The listing builds one solid part. Answer for the finished solid, in the listing's coordinates (mm). A direction names the side the tool comes from. Round coordinates to 2 decimals unless told otherwise and drop trailing zeros. Write each loop counter-clockwise with the first axis right and the second up, starting at its lowest first coordinate (ties: lowest second). Pieces come first, ordered by that corner, then holes.
Item 1: Find section B-B on y = 2.75. Give the vertices of the cut face in (x, z).
Item 2: Find the intervals of material crossed by probe 1 along X at (y, z) = (8.25, 0); probe 2 along Z at (x, y) = (-9.25, 2.75); probe 3 along Y at (x, z) = (9.75, 0), in increasing order.
Item 3: Find section C-C on z = -1.25. Give the vertices of the cut face in (x, y), then the cut area to 3 significant figures.
Item 4: Find section D-D on x = -10.5. Give the vertices of the cut face in (y, z), then the cut area to 3 significant figures.
Item 5: Find section A-A on x = 0. Give the vertices of the cut face in (y, z), then the cut area to 3 significant figures.
Item 6: A tool of negligible diameter and unlimited length cuts with its end or side. For faces 4 (the face through (-8, 5, 3)), 5 (the face through (8, 5, 3)), 6 (the face through (8, 5, -3)), 7 (the face through (0.1, 2.5, -2.5)), 8 (the face through (-8, 5, -3)), from which of +Z, -Z, +X, -X, +Y, -Y can it reach the whole face along a straight path? Write none if from no direction.
Item 7: For a pull along Y with two mould halves and no side action, classify faces 1 (the face through (-7.363, 4.485, 0.228)), 2 (the face through (-1, 7, 0)), 3 (the face through (0, 9.5, 2)) as +Y half, -Y half, draft (parallel to the pull), parting line (faces both ways), or undercut.
Item 8: Each of these flat-tipped pins is pushed along its axis until it touches: pin 1 (2 mm diameter, centred on x = -9, z = -3, fed in from -Y); pin 2 (4 mm diameter, centred on x = -9, y = 5, fed in from +Z); pin 3 (2.5 mm diameter, centred on x = 0, z = 0, fed in from -Y). Where does it stop, or does it pass through?
```python
from build123d import *

# Parameters (mm, degrees)
SKETCH1_R           = 4.7
SKETCH1_R_2         = 2.5
BOSS_EXTRUDE1_DEPTH = 5
SKETCH2_R           = 4.7
BOSS_EXTRUDE2_DEPTH = 4.5
SKETCH3_R           = 1
CUT_EXTRUDE1_DEPTH  = 4.5
SKETCH6_W           = 6
SKETCH6_H           = 6
BOSS_EXTRUDE3_DEPTH = 8.31
SKETCH7_W           = 6
SKETCH7_H           = 6
BOSS_EXTRUDE4_DEPTH = 2
FILLET1_R           = 1
BOSS_EXTRUDE5_DEPTH = 3
BOSS_EXTRUDE6_DEPTH = 9
FILLET2_R           = 1
SKETCH8_R           = 1.75
CUT_EXTRUDE6_DEPTH  = 37


with BuildPart() as part:
    # Sketch1 → Boss-Extrude1 (new body)
    with BuildSketch(Plane(origin=(0, 0, 0), x_dir=(1, 0, 0), z_dir=(0, 1, 0))):
        with Locations(Location((0, 0, 0), (0, 0, 270))):
            Circle(SKETCH1_R)
        with Locations(Location((0, 0, 0), (0, 0, 270))):
            Circle(SKETCH1_R_2, mode=Mode.SUBTRACT)
    extrude(amount=BOSS_EXTRUDE1_DEPTH)

    # Sketch2 → Boss-Extrude2 (add)
    with BuildSketch(Plane(origin=(0, 5, 0), x_dir=(1, 0, 0), z_dir=(0, 1, 0))):
        with Locations(Location((0, 0, 0), (0, 0, 270))):
            Circle(SKETCH2_R)
    extrude(amount=BOSS_EXTRUDE2_DEPTH)

    # Sketch3 → Cut-Extrude1 (cut)
    with BuildSketch(Plane(origin=(0, 9.5, 0), x_dir=(1, 0, 0), z_dir=(0, 1, 0))):
        with Locations(Location((0, 0, 0), (0, 0, 270))):
            Circle(SKETCH3_R)
    extrude(amount=-CUT_EXTRUDE1_DEPTH, mode=Mode.SUBTRACT)



with BuildPart() as body_2:
    # Sketch6 → Boss-Extrude3 (new body)
    with BuildSketch(Plane(origin=(4.7, 0, 0), x_dir=(0, 0, -1), z_dir=(1, 0, 0))):
        with Locations((0, 3.5)):
            Rectangle(SKETCH6_W, SKETCH6_H)
    extrude(amount=BOSS_EXTRUDE3_DEPTH)


with BuildPart() as part_1:
    add(part.part)

    add(body_2.part)  # Boss-Extrude4 merges body 2
    # Sketch7 → Boss-Extrude4 (add)
    with BuildSketch(Plane.ZY.offset(-4.7)):
        with Locations((0, 3.5)):
            Rectangle(SKETCH7_W, SKETCH7_H)
    extrude(amount=BOSS_EXTRUDE4_DEPTH)

    # Fillet1
    fillet1_edges = [part_1.edges().sort_by_distance(p)[0] for p in [
        (13.01, 3.5, -3),
        (13.01, 3.5, 3),
    ]]
    fillet(fillet1_edges, radius=FILLET1_R)

    # Sketch9 → Boss-Extrude5 (add)
    with BuildSketch(Plane(origin=(0, 6.5, 0), x_dir=(1, 0, 0), z_dir=(0, 1, 0))):
        with BuildLine():
            Line((13.01, -2), (13.01, 2))
            ThreePointArc((13.01, 2), (12.717106781, 2.707106781), (12.01, 3))
            Line((12.01, 3), (3.618010503, 3))
            ThreePointArc((3.618010503, 3), (4.7, 0), (3.618010503, -3))
            Line((3.618010503, -3), (12.01, -3))
            ThreePointArc((12.01, -3), (12.717106781, -2.707106781), (13.01, -2))
        make_face()
    extrude(amount=BOSS_EXTRUDE5_DEPTH)

    # Sketch10 → Boss-Extrude6 (add)
    with BuildSketch(Plane(origin=(0, 9.5, 0), x_dir=(1, 0, 0), z_dir=(0, 1, 0))):
        with BuildLine():
            Line((-13.1, -3), (-3.354101966, -3))
            ThreePointArc((-3.354101966, -3), (-4.5, 0), (-3.354101966, 3))
            Line((-3.354101966, 3), (-13.1, 3))
            Line((-13.1, 3), (-13.1, -3))
        make_face()
    extrude(amount=-BOSS_EXTRUDE6_DEPTH)

    # Fillet2
    fillet2_edges = [part_1.edges().sort_by_distance(p)[0] for p in [
        (-13.1, 5, -3),
        (-13.1, 5, 3),
    ]]
    fillet(fillet2_edges, radius=FILLET2_R)

    # Sketch8 → Cut-Extrude6 (cut)
    with BuildSketch(Plane(origin=(13.01, 0, 0), x_dir=(0, 0, -1), z_dir=(1, 0, 0))):
        with Locations((0, 2.75)):
            Circle(SKETCH8_R)
    extrude(amount=-CUT_EXTRUDE6_DEPTH, mode=Mode.SUBTRACT)


solid = part_1.part
```
Check values:
1. outline: (-13.1, -2) arc R1 ccw to (-12.1, -3) - (-3.62, -3) arc R4.7 ccw to (3.62, -3) - (12.01, -3) arc R1 ccw to (13.01, -2) - (13.01, -1.75) - (1.79, -1.75) arc R2.5 cw to (-1.79, -1.75) - (-13.1, -1.75) - close; (-13.1, 1.75) - (-1.79, 1.75) arc R2.5 cw to (1.79, 1.75) - (13.01, 1.75) - (13.01, 2) arc R1 ccw to (12.01, 3) - (3.62, 3) arc R4.7 ccw to (-3.62, 3) - (-12.1, 3) arc R1 ccw to (-13.1, 2) - close
2. probe 1: x = -13.1 to -1, 1 to 13.01
2. probe 2: z = -3 to -1.75, 1.75 to 3
2. probe 3: y = 0.5 to 1, 4.5 to 9.5
3. outline: (-13.1, 0.5) - (-4.53, 0.5) - (-4.53, 0) - (-2.17, 0) - (-2.17, 1.53) - (-13.1, 1.53) - close; (-13.1, 3.97) - (-2.17, 3.97) - (-2.17, 5) - (2.17, 5) - (2.17, 3.97) - (13.01, 3.97) - (13.01, 9.5) - (-13.1, 9.5) - close; (2.17, 0) - (4.53, 0) - (4.53, 0.5) - (13.01, 0.5) - (13.01, 1.53) - (2.17, 1.53) - close
3. area: 165 mm2
4. outline: (0.5, -3) - (9.5, -3) - (9.5, 3) - (0.5, 3) - close; hole circle Ø3.5 at (2.75, 0)
4. area: 44.4 mm2
5. outline: (0, -4.7) - (9.5, -4.7) - (9.5, -1) - (5, -1) - (5, -2.5) - (0, -2.5) - close; (0, 2.5) - (5, 2.5) - (5, 1) - (9.5, 1) - (9.5, 4.7) - (0, 4.7) - close
5. area: 55.3 mm2
6. face 4: +Z, -X, +Y, -Y
6. face 5: +Z, +X, +Y, -Y
6. face 6: -Z, +X, +Y, -Y
6. face 7: -Y
6. face 8: -Z, -X, +Y, -Y
7. face 1: undercut
7. face 2: draft
7. face 3: +Y half
8. pin 1: stops at y = 0.5
8. pin 2: stops at z = 3
8. pin 3: stops at y = 5
